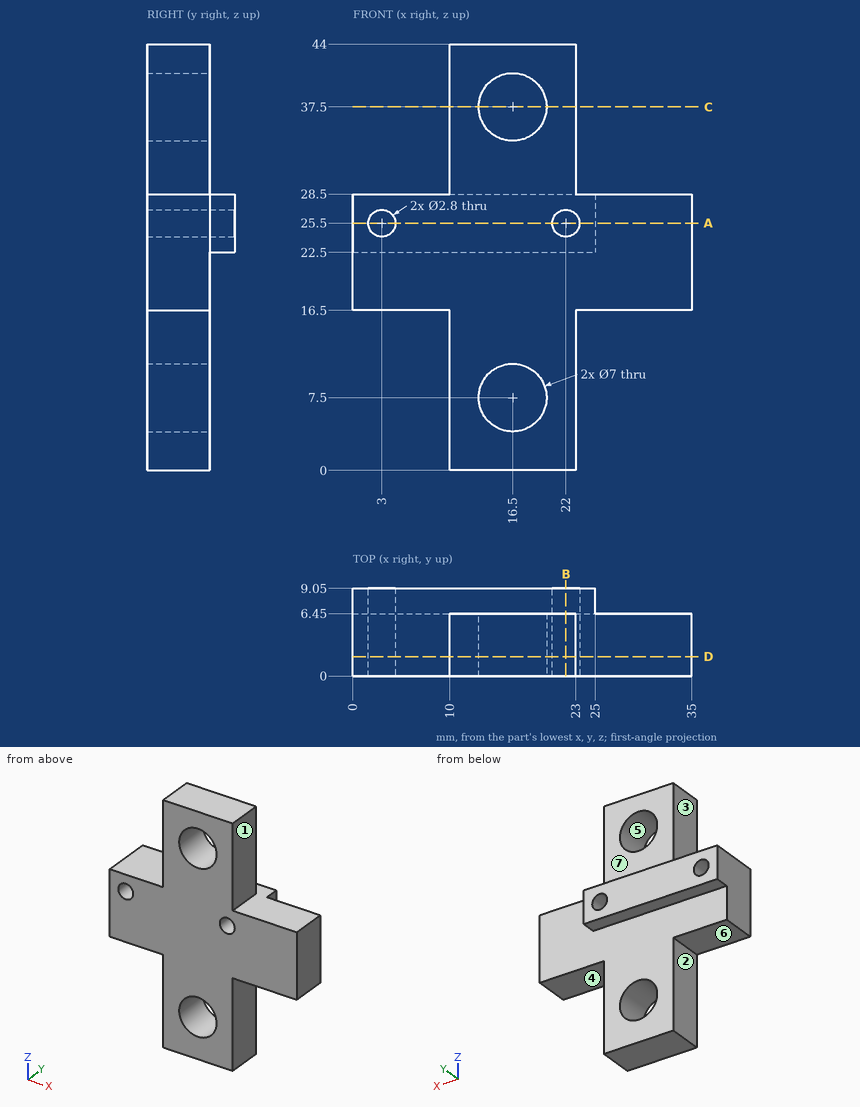
Source: three-view drawing plus pictorial views. Frame: mm from the lowest corner of the part. A direction names the side the tool comes from. Coordinates: 2 decimals unless noted, no trailing zeros. Order: outer loops, then holes, each group sorted by start corner. A loop starts at its lowest first (then second) coordinate and runs counter-clockwise, first axis right, second up.
Item 1: Cut plane C-C (z = 37.5). Return loops of the section in (x, y), plus the area to 3 significant figures.
Output values:
outline: (10, 0) - (13, 0) - (13, 6.45) - (10, 6.45) - close; (20, 0) - (23, 0) - (23, 6.45) - (20, 6.45) - close
area: 38.7 mm2
Item 2: Material intervals for line 1 (X direction, y = 4.25, z = 25.5); line 2 (Z direction, x = 16.5, y = 1.5); line 3 (X direction, y = 7, z = 25.5), sorted ascending.
Output values:
line 1: x = 0 to 1.6, 4.4 to 20.6, 23.4 to 35
line 2: z = 0 to 4, 11 to 34, 41 to 44
line 3: x = 0 to 1.6, 4.4 to 20.6, 23.4 to 25
Item 3: Pull-direction query (Z, two-part tool) for the marked faces 5, 6 and 7; classes: pulls with the +Z half, pulls with the -Z half, needs draft (parallel to the pull), parting line crosses it, or undercut.
Output values:
face 5: undercut
face 6: pulls with the -Z half
face 7: needs draft
Item 4: Set-up query: the marked faces 1, 2, 3 and 4. Return all of +Z, -Z, +X, -X, +Y, -Y with unobstructed straight access to the full face (end or side cutting, diameter ignored); none if empty.
Output values:
face 1: +Z, +X, +Y, -Y
face 2: -Z, -X, +Y, -Y
face 3: +Z, -X, +Y, -Y
face 4: -Z, +X, +Y, -Y
Item 5: Cut plane D-D (y = 2). Return loops of the section in (x, z).
Output values:
outline: (0, 16.5) - (10, 16.5) - (10, 0) - (23, 0) - (23, 16.5) - (35, 16.5) - (35, 28.5) - (23, 28.5) - (23, 44) - (10, 44) - (10, 28.5) - (0, 28.5) - close; hole circle Ø2.8 at (3, 25.5); hole circle Ø7 at (16.5, 7.5); hole circle Ø7 at (16.5, 37.5); hole circle Ø2.8 at (22, 25.5)
Item 6: First-contact query: P1, Ø2, axis at x = 14.5, y = 8, coming from the -Z side; P2, Ø4, axis at x = 18, z = 6.5, coming from the +Y side; P3, Ø2, axis at x = 3, z = 25.5, coming from the -Y side; P4, Ø1.9, axis at y = 4, z = 9.5, coming from the +X side. Flat tips, straight axial feed; report the tip coordinate or a pass-through.
Output values:
P1: stops at z = 22.5
P2: stops at y = 6.45
P3: passes through
P4: stops at x = 23
Item 7: Cut plane A-A (z = 25.5). Return loops of the section in (x, y).
Output values:
outline: (0, 0) - (1.6, 0) - (1.6, 9.05) - (0, 9.05) - close; (4.4, 0) - (20.6, 0) - (20.6, 9.05) - (4.4, 9.05) - close; (23.4, 0) - (35, 0) - (35, 6.45) - (25, 6.45) - (25, 9.05) - (23.4, 9.05) - close
Item 8: Cut plane B-B (x = 22). Return loops of the section in (y, z).
Output values:
outline: (0, 0) - (6.45, 0) - (6.45, 22.5) - (9.05, 22.5) - (9.05, 24.1) - (0, 24.1) - close; (0, 26.9) - (9.05, 26.9) - (9.05, 28.5) - (6.45, 28.5) - (6.45, 44) - (0, 44) - close
